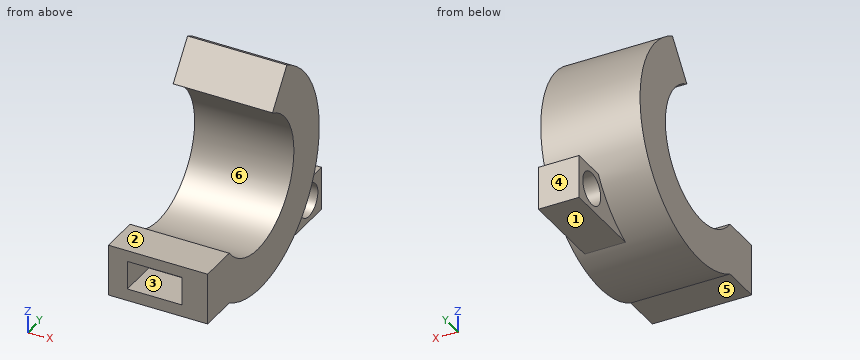
from build123d import *

# Parameters (mm, degrees)
F1_DEPTH = 15.494
F2_W     = 6.349988
F2_H     = 6.764519
F3_DEPTH = 13.208
F5_D     = 5.08
F6_W     = 15.494
F6_H     = 8.044068
F6_W_2   = 8.525903
F6_H_2   = 4.456614
F7_DEPTH = 6.1468


with BuildPart() as f1:
    # F0 (on Right) → F1 (new body)
    with BuildSketch(Plane.YZ):
        with BuildLine():
            ThreePointArc((-16.356304, 15.922897), (-12.415087, 0.19965), (-28.623536, 0))
            Line((-28.623536, 0), (-28.623536, -8.044068))
            ThreePointArc((-28.623536, -8.044068), (-5.189303, -1.794092), (-12.267232, 21.403503))
            Line((-12.267232, 21.403503), (-16.356304, 15.922897))
        make_face()
    extrude(amount=F1_DEPTH)

    # F2 (on Front) → F3 (join)
    with BuildSketch(Plane.XZ):
        with Locations((11.007179, -5.669695)):
            Rectangle(F2_W, F2_H)
    extrude(amount=F3_DEPTH)

    # F5 (through all)
    with Locations(Plane.YZ.offset(14.182173)):
        with Locations((-3.603312, -5.669695)):
            Hole(F5_D / 2)

    # F6 (on face) → F7 (join)
    with BuildSketch(Plane.XZ.offset(28.623536)):
        with Locations((7.747, -4.022034)):
            Rectangle(F6_W, F6_H)
        with Locations((7.216052, -3.949209)):
            Rectangle(F6_W_2, F6_H_2, mode=Mode.SUBTRACT)
    extrude(amount=F7_DEPTH)


solid = f1.part
Model file for the job. Use its own axes, mm. Face numbers are marked on the shaded views. A direction names the side the tool comes from. Coordinates: 2 decimals unless noted, no trailing zeros. Write each loop counter-clockwise with the first axis right and the second up, starting at its lowest first coordinate (ties: lowest second). Pieces come first, ordered by that corner, then holes. Notation, with made-up numbers: (13.5, 85) - (42.5, 85) arc R18 ccw to (42.5, 96) - close; hole circle Ø4 at (42.25, 29.25). An arc over 180 degrees is marked (long way). Write each question's results on one line, items separated by ' | '. Start each with the question number.
1) Cut at C-C (x = 4.5). Write the cut outline in (y, z), then the cut area to 3 significant figures.
2) Mould opens along Y. For the marked faces 4, 5 and 6 say: pulls with the +Y half, pulls with the -Y half, needs draft (parallel to the pull), parting line crosses it, or undercut.
3) 3-axis set-ups, long thin cutter, end or side, ignore diameter. For the marked faces 1, 2 and 3: which of +Z, -Z, +X, -X, +Y, -Y reach the whole face in a straight line?
4) Cut at A-A (y = -3.5). Write the cut outline in (x, z), then the cut area to 3 significant figures.
5) Cut at B-B (y = -31.5). Write the cut outline in (x, z), then the cut area to 3 significant figures.
6) Cut at D-D (x = 9.5). Write the cut outline in (y, z).
7) Probe line 1 along Z through (x, y) = (7.5, -30.5); line 2 along Y through (x, z) = (12.5, -5); line 3 along X through (y, z) = (-1.5, -8.5). List the from-to ranges inside material, lowest first. Write a range as from..to.
8) Flat gauge pins, fed straight in: P1, Ø5, axis at x = 7.5, z = 8, coming from the +Y side; P2, Ø6, axis at x = 11, y = -27.5, coming from the +Z side; P3, Ø6, axis at x = 12, y = -4, coming from the +Z side; P4, Ø18.5, axis at y = -20.6, z = 6.5, coming from the -X side. Where does each tip first touch, or does it go through?
Returned:
1) outline: (-34.77, -8.04) - (-28.62, -8.04) arc R16.85 ccw (long way) to (-12.27, 21.4) - (-16.36, 15.92) arc R10.33 cw (long way) to (-28.62, 0) - (-34.77, 0) - (-34.77, -1.72) - (-28.62, -1.72) - (-28.62, -6.18) - (-34.77, -6.18) - close | area: 337 mm^2
2) face 4: pulls with the +Y half | face 5: needs draft | face 6: undercut
3) face 1: -Z, +X, -X, +Y | face 2: +Z, +X, -X, -Y | face 3: -Y
4) outline: (0, 2.6) - (15.49, 2.6) - (15.49, 10.18) - (0, 10.18) - close; (7.83, -9.05) - (14.18, -9.05) - (14.18, -8.21) - (7.83, -8.21) - close; (7.83, -3.13) - (14.18, -3.13) - (14.18, -2.29) - (7.83, -2.29) - close | area: 128 mm^2
5) outline: (0, -8.04) - (15.49, -8.04) - (15.49, 0) - (0, 0) - close; hole (2.95, -6.18) - (11.48, -6.18) - (11.48, -1.72) - (2.95, -1.72) - close | area: 86.6 mm^2
6) outline: (-34.77, -8.04) - (-28.62, -8.04) arc R16.85 ccw to (-13.17, -9.05) - (0, -9.05) - (0, -2.29) - (-5.47, -2.29) arc R16.85 ccw to (-12.27, 21.4) - (-16.36, 15.92) arc R10.33 cw (long way) to (-28.62, 0) - (-34.77, 0) - (-34.77, -1.72) - (-28.62, -1.72) - (-28.62, -6.18) - (-34.77, -6.18) - close; hole circle Ø5.08 at (-3.6, -5.67)
7) line 1: -8.04..-6.18, -1.72..0 | line 2: -34.77..-6.05, -1.15..0 | line 3: 7.83..14.18
8) P1: y = -3.07 | P2: z = 0 | P3: z = 17.21 | P4: through
